Geometry: final body of the model. Coordinates: model frame, mm. Face numbers are marked on the shaded views. A direction names the side the tool comes from. Give positions to 0.01 mm unless a question says otherwise; leave off trailing zeros. Write each loop counter-clockwise with the first axis right and the second up, starting at its lowest first coordinate (ties: lowest second). Pieces come first, ordered by that corner, then holes. Notation, with made-up numbers: (17, -21.5) - (51, -21.5) arc R9 cw to (51, -11.5) - close; hole circle Ø1 at (42.5, -32.75). An arc over 180 degrees is marked (long way). Return JSON: item names as keys, results as strings.
from build123d import *


with BuildPart() as f1:
    # F0 (on Front) → F1 (revolve)
    with BuildSketch(Plane.XZ):
        with BuildLine():
            Line((24, 84), (0, 84))
            Line((0, 84), (-24, 84))
            Line((-24, 84), (-24, 67.5))
            Line((-24, 67.5), (-14, 67.5))
            ThreePointArc((-14, 67.5), (-12.585786, 66.914214), (-12, 65.5))
            Line((-12, 65.5), (-12, 46))
            ThreePointArc((-12, 46), (-12.585786, 44.585786), (-14, 44))
            Line((-14, 44), (-24, 44))
            Line((-24, 44), (-24, 34))
            Line((-24, 34), (-21, 34))
            Line((-21, 34), (-21, 35.5))
            Line((-21, 35.5), (-18, 35.5))
            Line((-18, 35.5), (-18, 34))
            Line((-18, 34), (-3, 34))
            Line((-3, 34), (-3, 30))
            Line((-3, 30), (0, 30))
            Line((0, 30), (3, 30))
            Line((3, 30), (3, 34))
            Line((3, 34), (18, 34))
            Line((18, 34), (18, 35.5))
            Line((18, 35.5), (21, 35.5))
            Line((21, 35.5), (21, 34))
            Line((21, 34), (24, 34))
            Line((24, 34), (24, 44))
            Line((24, 44), (14, 44))
            ThreePointArc((14, 44), (12.585786, 44.585786), (12, 46))
            Line((12, 46), (12, 65.5))
            ThreePointArc((12, 65.5), (12.585786, 66.914214), (14, 67.5))
            Line((14, 67.5), (24, 67.5))
            Line((24, 67.5), (24, 84))
        make_face()
    revolve(axis=Axis((-12, 0, 0), (1, 0, 0)))


solid = f1.part
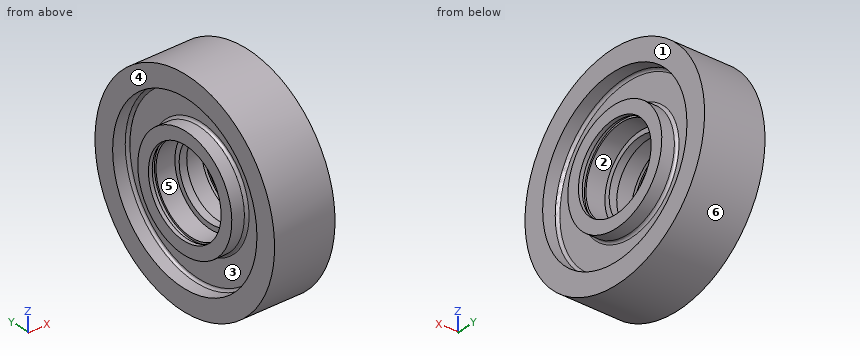
Q1. Set-up query: the marked faces 1, 2 and 3. Return all of +Z, -Z, +X, -X, +Y, -Y with unobstructed straight access to the full face (end or side cutting, diameter ignored); none if empty.
Answer key:
{"face 1": "+Z, -Z, +X, +Y, -Y", "face 2": "+X", "face 3": "-X"}
Q2. Material intervals for probe 1 along Y at (x, z) = (19, 0); probe 2 along Y at (x, z) = (-21.5, 0), sorted ascending. Write a range as [from, to].
Answer key:
{"probe 1": "y = [-84, -67.5], [-44, -35.5], [35.5, 44], [67.5, 84]", "probe 2": "y = [-84, -67.5], [-44, -34], [34, 44], [67.5, 84]"}
Q3. Pin query (flat end, axial travel): P1, Ø12, axis at x = 7, z = -14.5, coming from the +Y side; P2, Ø4, axis at y = -31.5, z = -40.5, coming from the +X side; P3, Ø12, axis at x = -10.5, z = -13.5, coming from the -Y side. Return the tip coordinate at first contact, or that it passes through.
Answer key:
{"P1": "stops at y = 83.57", "P2": "stops at x = 12", "P3": "stops at y = -83.66"}
Q4. Mould query, pull axis Z, two halves, no side actions, for the marked faces 4, 5 and 6. Classes: pulls with the +Z half, pulls with the -Z half, needs draft (parallel to the pull), parting line crosses it, or undercut.
Answer key:
{"face 4": "needs draft", "face 5": "undercut", "face 6": "parting line crosses it"}
Q5. Section query B-B, the plane y = -72. Return the cut outline in (x, z).
Answer key:
{"outline": "(-24, -43.27) - (24, -43.27) - (24, 43.27) - (-24, 43.27) - close"}
Q6. Section query A-A, the plane x = 16. Return the cut outline in (y, z).
Answer key:
{"outline": "circle Ø168 at (0, 0); circle Ø88 at (0, 0); hole circle Ø135 at (0, 0); hole circle Ø68 at (0, 0)"}
